Autodesk Inventor part; units mm, degrees
ref_plane "XZ Plane" through (0, 0, 0) normal (0, 1, 0) x (-1, 0, 0)
sketch "Sketch1" plane through (0, 0, 0) normal (0, 1, 0) x (-1, 0, 0)
  circle A0 centre (0, 0) radius 4
  dimension "d0" = 8
extrude "Extrusion1" add sketch "Sketch1" along normal blind 1
sketch "Sketch2" plane through (0, 1, 0) normal (0, 1, 0) x (1, 0, 0)
  circle A0 centre (0, 0) radius 4
  circle A1 centre (0, 0) radius 3
  dimension "d3" = 6
extrude "Extrusion2" add sketch "Sketch2" along normal blind 15.668 contours A1
sketch "Sketch3" plane through (0, 0, 0) normal (0, -1, 0) x (1, 0, 0)
  circle A0 centre (0, 0) radius 4
  circle A1 centre (0, 0) radius 1
  dimension "d6" = 2
extrude "Extrusion3" cut sketch "Sketch3" against normal blind 21 contours A1
sketch "Sketch4" plane through (0, 0, 0) normal (1, 0, 0) x (0, 1, 0)
  line L0 (1, 3) -> (16.668, 3)
  line L1 (1, -3) -> (16.668, -3)
  line L2 (0, 0) -> (17, 0)
  line L3 (16.668, 3) -> (18.9755, 0.25)
  line L4 (16.668, -3) -> (16.668, 3)
  line L5 (16.668, 0.2) -> (18.9755, 0.2)
  line L6 (17.7072, 0.4) -> (16.668, 1)
  line L7 (0, 1) -> (16.668, 1)
  line L8 (16.668, 1) -> (16.668, 3)
  line L9 (18.9755, 0.25) -> (18.9755, 0.2)
  line L10 (17.7072, 0.4) -> (18.8077, 0.4)
  line L11 (18.8077, 0.4) -> (18.8077, 0.45)
  point P0 (17.8856, 0.2)
  dimension "d9" = 40
  dimension "d10" = 0.2
  dimension "d11" = 30
  dimension "d20" = 0.05
  dimension "d21" = 0.4
  dimension "d22" = 0.05
revolve "Revolution1" add sketch "Sketch4" angle 360 about axis through (0, 0, 0) along (0, 1, 0) contours L3 L11 L10 L6 L4
sketch "Sketch5" plane through (0, 0, 0) normal (0, 0, 1) x (1, 0, 0)
  circle A0 centre (3, 1.35) radius 0.35
  line L0 (4, 1) -> (-4, 1)
  line L1 (3, 3) -> (3, 0)
  line L2 (0, 1.1204) -> (0, 3)
  line L3 (2.7525, 1.5975) -> (3.3734, 2.2184)
  line L4 (3.3734, 2.2184) -> (3.3499, 1.3406)
  point P0 (0, 0)
  dimension "d14" = 0.7
  dimension "d19" = 45
revolve "Revolution2" cut sketch "Sketch5" angle 360 about axis through (0, 1.1204, 0) along (0, 1, 0)
chamfer "Chamfer1" distance 0.3 angle 45 1 edges at (4, 1, 0)
sketch "Sketch6" plane through (0, 0, 0) normal (0, 0, 1) x (1, 0, 0)
  line L0 (-3, 1.845) -> (-3, 16.668)
  line L1 (-3, 3) -> (-2.4, 3)
  line L2 (-2.4, 3) -> (-2.4, 4)
  line L3 (-2.4, 4) -> (-3, 4)
  line L4 (-3, 4) -> (-3, 3)
  line L5 (-4, 0) -> (4, 0)
  line L6 (0, 0) -> (0, -2.0894)
  dimension "d23" = 0.6
  dimension "d24" = 1
  dimension "d25" = 3
revolve "Revolution3" cut sketch "Sketch6" angle 360 about axis through (0, 0, 0) along (0, -1, 0)
properties part number "nozzle0.8" material "Copper"
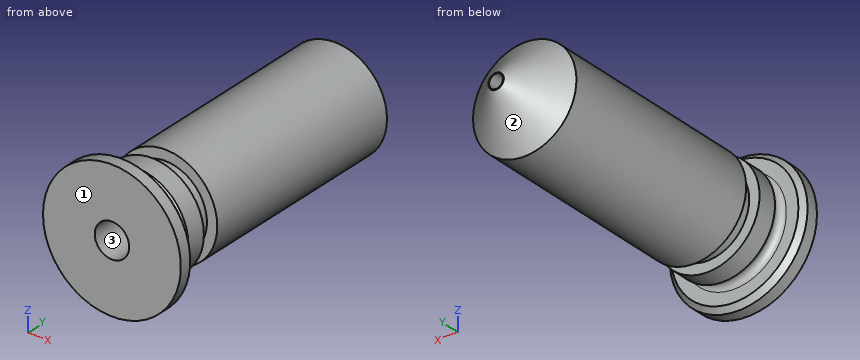
Model file for the job. Use its own axes, mm. Face numbers are marked on the shaded views. Round coordinates to 2 decimals unless told otherwise and drop trailing zeros. Loops run counter-clockwise (first coordinate to the right, second up) from the corner with the lowest first, then second, coordinate; pieces in that order, holes last.
1. Wall check: probe 1 along X at (y, z) = (3.5, 0); probe 2 along Y at (x, z) = (-1.25, -2.5); probe 3 along X at (y, z) = (7.75, 0). Give the ranges that are in metal, low to high.
Check values:
probe 1: x = -2.4 to -1, 1 to 2.4
probe 2: y = 0 to 1.07, 1.64 to 3, 4 to 16.84
probe 3: x = -3 to -1, 1 to 3
2. Mould opens along Z. For the marked faces 1, 2 and 3 say: +Z half, -Z half, draft (parallel to the pull), parting line (faces both ways), or undercut.
Check values:
face 1: draft
face 2: parting line
face 3: undercut
3. Band-saw the part on C-C, the plane y = 9. List the corners of the cut face in (x, z), and give its area (3 significant figures).
Check values:
outline: circle Ø6 at (0, 0); hole circle Ø2 at (0, 0)
area: 25.1 mm2
4. Drop flat-ended pins along their axis: P1, Ø4, axis at x = 1.5, y = 12, coming from the -Z side; P2, Ø1, axis at y = 12.5, z = 1, coming from the -X side; P3, Ø3, axis at x = 1.5, y = 15, coming from the +Z side. Give the stop position or say it passes through.
Check values:
P1: stops at z = -3
P2: stops at x = -2.96
P3: stops at z = 3
5. Band-saw the part on D-D, the plane z = 2.75. Count the separate pieces of the cut face and the enclosed holes in it, and give its area (3 significant figures).
Check values:
separate pieces: 3
enclosed holes: 0
area: 39.7 mm2
